```python
from build123d import *

# Parameters (mm, degrees)
SKETCH_1_W          = 114
SKETCH_1_H          = 68
EXTRUDE_1_DEPTH     = 1
CUT_EXTRUDE_1_REACH = 3
SKETCH_2_R          = 2.25


with BuildPart() as part:
    # Эскиз1 → Бобышка-Вытянуть1 (new body)
    with BuildSketch(Plane.XY):
        with Locations((57, 34)):
            Rectangle(SKETCH_1_W, SKETCH_1_H)
    extrude(amount=EXTRUDE_1_DEPTH)

    # Эскиз2 → Вырез-Вытянуть1 (cut, up to next)
    with BuildSketch(Plane.XY.offset(1), mode=Mode.PRIVATE) as cut_extrude_1_sk1:
        with Locations((6, 62)):
            Circle(SKETCH_2_R)
    cut_extrude_1_tool1 = extrude(cut_extrude_1_sk1.sketch, amount=-CUT_EXTRUDE_1_REACH, mode=Mode.PRIVATE) & part.part
    add(cut_extrude_1_tool1.solids().sort_by_distance((6, 62, 1))[0], mode=Mode.SUBTRACT)
    # Эскиз2 → Вырез-Вытянуть1 (cut, up to next)
    with BuildSketch(Plane.XY.offset(1), mode=Mode.PRIVATE) as cut_extrude_1_sk2:
        with Locations((6, 28)):
            Circle(SKETCH_2_R)
    cut_extrude_1_tool2 = extrude(cut_extrude_1_sk2.sketch, amount=-CUT_EXTRUDE_1_REACH, mode=Mode.PRIVATE) & part.part
    add(cut_extrude_1_tool2.solids().sort_by_distance((6, 28, 1))[0], mode=Mode.SUBTRACT)
    # Эскиз2 → Вырез-Вытянуть1 (cut, up to next)
    with BuildSketch(Plane.XY.offset(1), mode=Mode.PRIVATE) as cut_extrude_1_sk3:
        with Locations((6, 6)):
            Circle(SKETCH_2_R)
    cut_extrude_1_tool3 = extrude(cut_extrude_1_sk3.sketch, amount=-CUT_EXTRUDE_1_REACH, mode=Mode.PRIVATE) & part.part
    add(cut_extrude_1_tool3.solids().sort_by_distance((6, 6, 1))[0], mode=Mode.SUBTRACT)
    # Эскиз2 → Вырез-Вытянуть1 (cut, up to next)
    with BuildSketch(Plane.XY.offset(1), mode=Mode.PRIVATE) as cut_extrude_1_sk4:
        with Locations((57, 6)):
            Circle(SKETCH_2_R)
    cut_extrude_1_tool4 = extrude(cut_extrude_1_sk4.sketch, amount=-CUT_EXTRUDE_1_REACH, mode=Mode.PRIVATE) & part.part
    add(cut_extrude_1_tool4.solids().sort_by_distance((57, 6, 1))[0], mode=Mode.SUBTRACT)
    # Эскиз2 → Вырез-Вытянуть1 (cut, up to next)
    with BuildSketch(Plane.XY.offset(1), mode=Mode.PRIVATE) as cut_extrude_1_sk5:
        with Locations((57, 62)):
            Circle(SKETCH_2_R)
    cut_extrude_1_tool5 = extrude(cut_extrude_1_sk5.sketch, amount=-CUT_EXTRUDE_1_REACH, mode=Mode.PRIVATE) & part.part
    add(cut_extrude_1_tool5.solids().sort_by_distance((57, 62, 1))[0], mode=Mode.SUBTRACT)
    # Эскиз2 → Вырез-Вытянуть1 (cut, up to next)
    with BuildSketch(Plane.XY.offset(1), mode=Mode.PRIVATE) as cut_extrude_1_sk6:
        with Locations((108, 62)):
            Circle(SKETCH_2_R)
    cut_extrude_1_tool6 = extrude(cut_extrude_1_sk6.sketch, amount=-CUT_EXTRUDE_1_REACH, mode=Mode.PRIVATE) & part.part
    add(cut_extrude_1_tool6.solids().sort_by_distance((108, 62, 1))[0], mode=Mode.SUBTRACT)
    # Эскиз2 → Вырез-Вытянуть1 (cut, up to next)
    with BuildSketch(Plane.XY.offset(1), mode=Mode.PRIVATE) as cut_extrude_1_sk7:
        with Locations((108, 28)):
            Circle(SKETCH_2_R)
    cut_extrude_1_tool7 = extrude(cut_extrude_1_sk7.sketch, amount=-CUT_EXTRUDE_1_REACH, mode=Mode.PRIVATE) & part.part
    add(cut_extrude_1_tool7.solids().sort_by_distance((108, 28, 1))[0], mode=Mode.SUBTRACT)
    # Эскиз2 → Вырез-Вытянуть1 (cut, up to next)
    with BuildSketch(Plane.XY.offset(1), mode=Mode.PRIVATE) as cut_extrude_1_sk8:
        with Locations((108, 6)):
            Circle(SKETCH_2_R)
    cut_extrude_1_tool8 = extrude(cut_extrude_1_sk8.sketch, amount=-CUT_EXTRUDE_1_REACH, mode=Mode.PRIVATE) & part.part
    add(cut_extrude_1_tool8.solids().sort_by_distance((108, 6, 1))[0], mode=Mode.SUBTRACT)
    # Эскиз2 → Вырез-Вытянуть1 (cut, up to next)
    with BuildSketch(Plane.XY.offset(1), mode=Mode.PRIVATE) as cut_extrude_1_sk9:
        with BuildLine():
            Line((59, 36.368871126), (59, 31.4))
            ThreePointArc((59, 31.4), (57, 29.4), (55, 31.4))
            Line((55, 31.4), (55, 36.368871126))
            ThreePointArc((55, 36.368871126), (57, 44.9), (59, 36.368871126))
        make_face()
    cut_extrude_1_tool9 = extrude(cut_extrude_1_sk9.sketch, amount=-CUT_EXTRUDE_1_REACH, mode=Mode.PRIVATE) & part.part
    add(cut_extrude_1_tool9.solids().sort_by_distance((57, 38.298039, 1))[0], mode=Mode.SUBTRACT)


solid = part.part
```
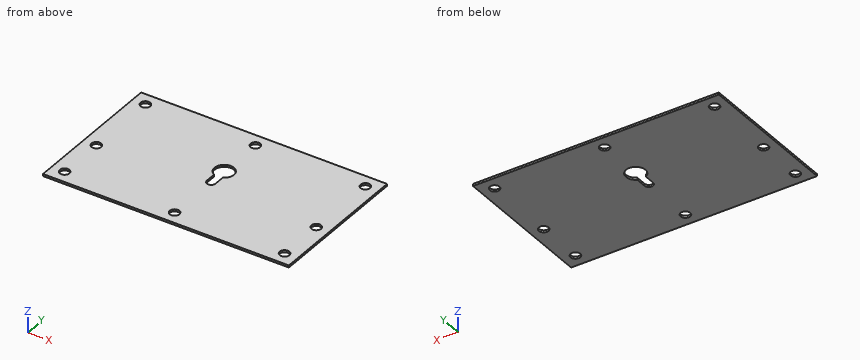
Read the model definition and answer for the solid it produces. Units are mm, in the model's axes. Give positions to 0.01 mm unless a question says otherwise; leave off trailing zeros. Order: outer loops, then holes, each group sorted by start corner. A loop starts at its lowest first (then second) coordinate and runs counter-clockwise, first axis right, second up. Notation, with made-up numbers: (72, 2.5) -> (96, 2.5) arc R13 cw to (96, 20.5) -> close; hole circle Ø6 at (-25.5, 83). An arc over 180 degrees is marked (long way). One line per item, written item: value. Start each with the question number.
(1) The part is cut by section B-B (x = 57). Determine the outline of the cut face in (y, z), and give its area (3 significant figures).
(2) A flat-ended cylindrical pin translates along its axis: P1, Ø8, axis at x = 57, y = 40.4, coming from the +Z side. Find the tip coordinate at first contact, or state that the pin passes through.
(3) The part is cut by section A-A (z = 0.55). State how many separate pieces and enclosed holes the cut face has, and give its area (3 significant figures).
(4) The part is cut by section D-D (y = 40.4). Determine the outline of the cut face in (x, z).
(5) The part is cut by section C-C (y = 28). Determine the outline of the cut face in (x, z).
(6) Straight lines are drawn through the part: L1, parallel to Y at x = 57, z = 0.2; L2, parallel to X at y = 40.4, z = 0.2; L3, parallel to X at y = 36, z = 0.7. For each, find the intervals that lie inside material, in ascending order.
Taken from the geometry:
1. outline: (0, 0) -> (3.75, 0) -> (3.75, 1) -> (0, 1) -> close; (8.25, 0) -> (29.4, 0) -> (29.4, 1) -> (8.25, 1) -> close; (44.9, 0) -> (59.75, 0) -> (59.75, 1) -> (44.9, 1) -> close; (64.25, 0) -> (68, 0) -> (68, 1) -> (64.25, 1) -> close
1. area: 43.5 mm^2
2. P1: through
3. separate pieces: 1
3. enclosed holes: 9
3. area: 7,540 mm^2
4. outline: (0, 0) -> (52.5, 0) -> (52.5, 1) -> (0, 1) -> close; (61.5, 0) -> (114, 0) -> (114, 1) -> (61.5, 1) -> close
5. outline: (0, 0) -> (3.75, 0) -> (3.75, 1) -> (0, 1) -> close; (8.25, 0) -> (105.75, 0) -> (105.75, 1) -> (8.25, 1) -> close; (110.25, 0) -> (114, 0) -> (114, 1) -> (110.25, 1) -> close
6. L1: 0 to 3.75, 8.25 to 29.4, 44.9 to 59.75, 64.25 to 68
6. L2: 0 to 52.5, 61.5 to 114
6. L3: 0 to 55, 59 to 114
